from build123d import *

# Parameters (mm, degrees)
BLANKSKE_W                   = 100
BLANKSKE_H                   = 11.5
BLANK_DEPTH                  = 5
TOOTHCUTSIM_DEPTH            = 101.783183121
TEETHCUTS_COUNT              = 22
TEETHCUTS_PITCH              = 4.712388975
BOSS_EXTRU_1_DEPTH           = 5
BOSS_EXTRU_2_DEPTH           = 5
CONG_2_R                     = 2.5
CONG_3_R                     = 2.5
CONG_4_R                     = 2.5
ENL_V_MAT_EXTRU_1_DEPTH      = 116.139334748
ENL_V_MAT_EXTRU_1_DEPTH_BACK = 116.139334748
ESQUISSE4_W                  = 53.825648792
ESQUISSE4_H                  = 17.774257486
BOSS_EXTRU_3_DEPTH           = 5


with BuildPart() as part:
    # BlankSke → Blank (new body)
    with BuildSketch(Plane.XY):
        with Locations((50, 5.75)):
            Rectangle(BLANKSKE_W, BLANKSKE_H)
    extrude(amount=-BLANK_DEPTH)

    # TooCutSkeSim → ToothCutSim (cut, through all)
    with BuildSketch(Plane.XY):
        Polygon((0.654653055, 8.125), (-0.654653055, 8.125), (-1.892297439, 11.5254), (1.892297439, 11.5254), align=None)
    toothcutsim = extrude(amount=-TOOTHCUTSIM_DEPTH, mode=Mode.SUBTRACT)

    # TeethCuts: ToothCutSim ×22
    with Locations(*[(i * TEETHCUTS_PITCH, 0, 0) for i in range(1, TEETHCUTS_COUNT)]):
        add(toothcutsim, mode=Mode.SUBTRACT)

    # Esquisse1 → Boss.-Extru.1 (add)
    with BuildSketch(Plane(origin=(100, 0, 0), x_dir=(0, 0, -1), z_dir=(1, 0, 0))):
        with BuildLine():
            Line((5, 12.18326915), (0, 12.18326915))
            ThreePointArc((0, 12.18326915), (-2.121320344, 11.304589494), (-3, 9.18326915))
            Line((-3, 9.18326915), (-3, 0))
            ThreePointArc((-3, 0), (-2.121320344, -2.121320344), (0, -3))
            Line((0, -3), (5, -3))
            ThreePointArc((5, -3), (7.121320344, -2.121320344), (8, 0))
            Line((8, 0), (8, 9.18326915))
            ThreePointArc((8, 9.18326915), (7.121320344, 11.304589494), (5, 12.18326915))
        make_face()
    extrude(amount=BOSS_EXTRU_1_DEPTH)

    # Esquisse2 → Boss.-Extru.2 (add)
    with BuildSketch(Plane.ZY):
        with BuildLine():
            Line((-5, 46.5625), (0, 46.5625))
            ThreePointArc((0, 46.5625), (1.767766953, 45.830266953), (2.5, 44.0625))
            Line((2.5, 44.0625), (2.5, -35.9375))
            ThreePointArc((2.5, -35.9375), (1.767766953, -37.705266953), (0, -38.4375))
            Line((0, -38.4375), (-5, -38.4375))
            ThreePointArc((-5, -38.4375), (-6.767766953, -37.705266953), (-7.5, -35.9375))
            Line((-7.5, -35.9375), (-7.5, 44.0625))
            ThreePointArc((-7.5, 44.0625), (-6.767766953, 45.830266953), (-5, 46.5625))
        make_face()
    extrude(amount=BOSS_EXTRU_2_DEPTH)

    # Congé2
    cong_2_edges = [part.edges().sort_by_distance(p)[0] for p in [
        (0, 4.0625, -5),
    ]]
    fillet(cong_2_edges, radius=CONG_2_R - 0.0001)  # a hair under: the kernel refuses the full size

    # Congé3
    cong_3_edges = [part.edges().sort_by_distance(p)[0] for p in [
        (0, 4.0625, 0),
    ]]
    fillet(cong_3_edges, radius=CONG_3_R - 0.0001)  # a hair under: the kernel refuses the full size

    # Congé4
    cong_4_edges = [part.edges().sort_by_distance(p)[0] for p in [
        (0, 0, -2.5),
    ]]
    fillet(cong_4_edges, radius=CONG_4_R)

    # Esquisse4 → Enlèv. mat.-Extru.1 (cut, two sides: drawn at the far end of the back side and taken through both)
    with BuildSketch(Plane(origin=(0, 0, -5), x_dir=(-1, 0, 0), z_dir=(0, 0, -1)).offset(-ENL_V_MAT_EXTRU_1_DEPTH_BACK)):
        with Locations((-78.087175604, 5.887128743)):
            Rectangle(ESQUISSE4_W, ESQUISSE4_H)
    extrude(amount=ENL_V_MAT_EXTRU_1_DEPTH + ENL_V_MAT_EXTRU_1_DEPTH_BACK, mode=Mode.SUBTRACT)

    # Esquisse5 → Boss.-Extru.3 (add)
    with BuildSketch(Plane(origin=(51.174351208, 0, 0), x_dir=(0, 0, -1), z_dir=(1, 0, 0))):
        with BuildLine():
            Line((0, 14.07249321), (5, 14.07249321))
            ThreePointArc((5, 14.07249321), (6.767766953, 13.340260163), (7.5, 11.57249321))
            Line((7.5, 11.57249321), (7.5, -3.42750679))
            ThreePointArc((7.5, -3.42750679), (6.767766953, -5.195273743), (5, -5.92750679))
            Line((5, -5.92750679), (0, -5.92750679))
            ThreePointArc((0, -5.92750679), (-1.767766953, -5.195273743), (-2.5, -3.42750679))
            Line((-2.5, -3.42750679), (-2.5, 11.57249321))
            ThreePointArc((-2.5, 11.57249321), (-1.767766953, 13.340260163), (0, 14.07249321))
        make_face()
    extrude(amount=BOSS_EXTRU_3_DEPTH)


solid = part.part
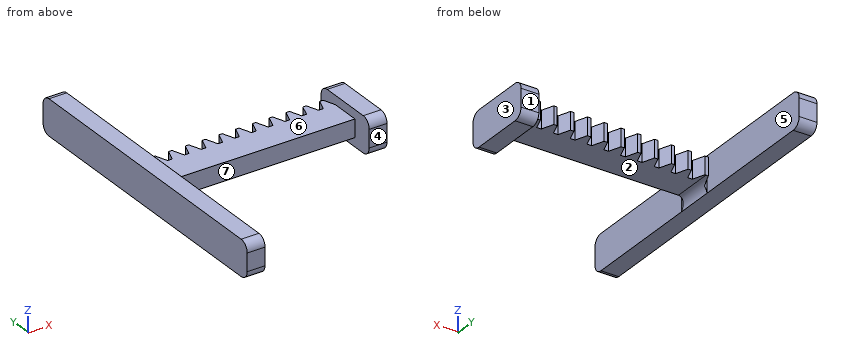
The listing builds one solid part. Answer for the finished solid, in the listing's coordinates (mm). Face numbers are marked on the shaded views. A direction names the side the tool comes from. Give positions to 0.01 mm unless a question says otherwise; leave off trailing zeros. Order: outer loops, then holes, each group sorted by start corner. A loop starts at its lowest first (then second) coordinate and runs counter-clockwise, first axis right, second up. Notation, with made-up numbers: (15, -16.5) -> (19, -16.5) arc R24 ccw to (19, 8.5) -> close; hole circle Ø4 at (70.25, -3.5). An arc over 180 degrees is marked (long way). Put each result on its own line as item: value.
Item 1: Straight lines are drawn through the part: line 1 (X direction, y = 12.5, z = -3.25); line 2 (X direction, y = -6, z = -7); line 3 (Y direction, x = 33.5, z = -2.75) (3 decimals). For each, find the intervals that lie inside material, in ascending order.
Established:
line 1: x = -5 to 0, 51.17 to 56.17
line 2: x = -5 to 0
line 3: y = 0 to 8.125
Item 2: For a pull along X with two mould halves and no side action, classify the marked faces 1, 2 and 3 as released by +X, released by -X, zero draft, split by the parting line, or undercut.
Established:
face 1: zero draft
face 2: undercut
face 3: released by +X
Item 3: For the marked faces 4, 5, 6 and 7, determine the directions among +Z, -Z, +X, -X, +Y, -Y from which every point of the face is accessible in a straight line to the end or side of a thin tool.
Established:
face 4: +Z, -Z, +X, -Y
face 5: +Z, -Z
face 6: +Z, +Y, -Y
face 7: +Z, -Z, -Y
Item 4: Given P1, Ø5, axis at y = 33, z = 1, coming from the +X side; P2, Ø0.8, axis at x = 7, z = -2, coming from the +Y side; P3, Ø5, axis at x = 43, z = -1, coming from the -Y side; P4, Ø8, axis at x = 7.5, y = -28.5, coming from the -Z side, each flat-ended and moving along its own axis, determine where each tip first touches the part or whether it passes through.
Established:
P1: stops at x = 0
P2: stops at y = 11.5
P3: stops at y = 0
P4: passes through
Item 5: A cutting plane is placed at B-B on y = 39. Give the vertices of the cut face in (x, z), plus the area to 3 significant figures.
Established:
outline: (-5, -7.5) -> (0, -7.5) -> (0, 2.5) -> (-5, 2.5) -> close
area: 50.0 mm^2
